Print and shaded views of the part. All mm, measured from the part's lowest x, y and z. A direction names the side the tool comes from. Coordinates: 2 decimals unless noted, no trailing zeros. Loops run counter-clockwise (first coordinate to the right, second up) from the corner with the lowest first, then second, coordinate; pieces in that order, holes last. Notation, with made-up numbers: (19, 18.25) -> (32, 18.25) arc R28 ccw to (32, 43.25) -> close; hole circle Ø3 at (40.5, 83). An arc over 180 degrees is marked (long way). One line per question, with ' | ' between items. Start each with the question number.
1) Cut at A-A (x = 622.5). List the corners of the cut face in (y, z) (1 decimal), plus the area to 3 significant figures.
2) Probe L1, parallel to Y at x = 335, z = 46 (1 decimal); L2, parallel to X at y = 92.5, z = 75 (1 decimal); L3, parallel to Z at x = 325, y = 17. List the from-to ranges inside material, lowest first. Write a range as from..to.
3) Cut at C-C (z = 47.5). List the corners of the cut face in (x, y) (1 decimal), plus the area to 3 significant figures.
4) 3-axis set-ups, long thin cutter, end or side, ignore diameter. For the marked faces 1 and 2: which of +Z, -Z, +X, -X, +Y, -Y reach the whole face in a straight line?
5) Cut at B-B (y = 56.5). List the corners of the cut face in (x, z) (1 decimal), plus the area to 3 significant figures.
6) Drop flat-ended pins along their axis: pin 1 (21.5 mm diameter, centred on x = 555.5, z = 64.5, fed in from +Y) (1 decimal); pin 2 (2 mm diameter, centred on x = 546.5, z = 35.5, fed in from -Y); pin 3 (1 mm diameter, centred on y = 51, z = 39, fed in from -X). Give the stop position or say it passes through.
7) Cut at D-D (y = 148). List the corners of the cut face in (x, z).
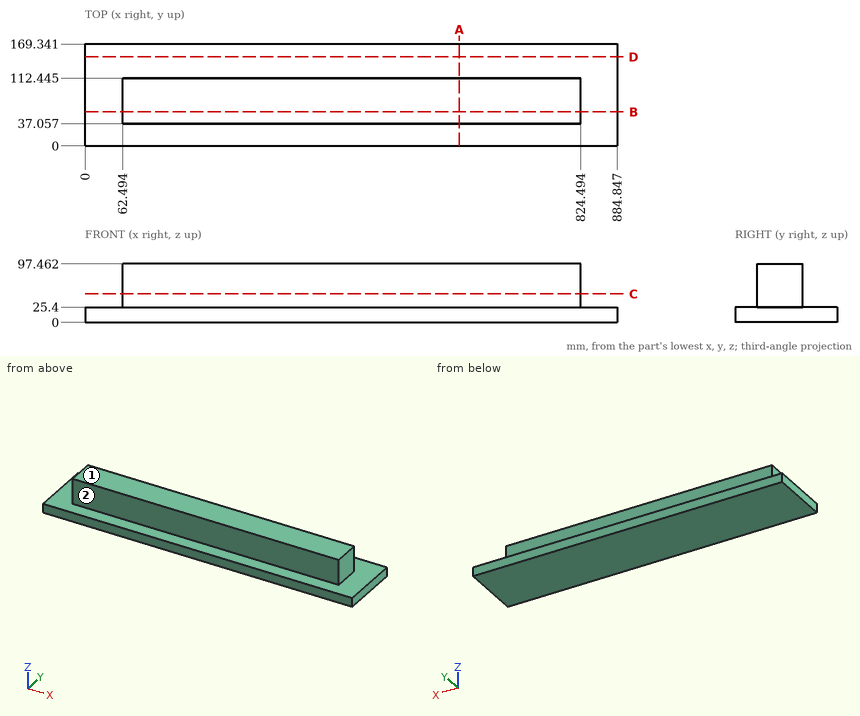
Reported:
1) outline: (0, 0) -> (169.3, 0) -> (169.3, 25.4) -> (112.4, 25.4) -> (112.4, 97.5) -> (37.1, 97.5) -> (37.1, 25.4) -> (0, 25.4) -> close | area: 9,730 mm²
2) L1: y = 37.1..112.4 | L2: x = 62.5..824.5 | L3: z = 0..25.4
3) outline: (62.5, 37.1) -> (824.5, 37.1) -> (824.5, 112.4) -> (62.5, 112.4) -> close | area: 57,400 mm²
4) face 1: +Z, +X, -X, +Y, -Y | face 2: +Z, +X, -X, -Y
5) outline: (0, 0) -> (884.8, 0) -> (884.8, 25.4) -> (824.5, 25.4) -> (824.5, 97.5) -> (62.5, 97.5) -> (62.5, 25.4) -> (0, 25.4) -> close | area: 77,400 mm²
6) pin 1: stops at y = 112.4 | pin 2: stops at y = 37.06 | pin 3: stops at x = 62.49
7) outline: (0, 0) -> (884.85, 0) -> (884.85, 25.4) -> (0, 25.4) -> close
